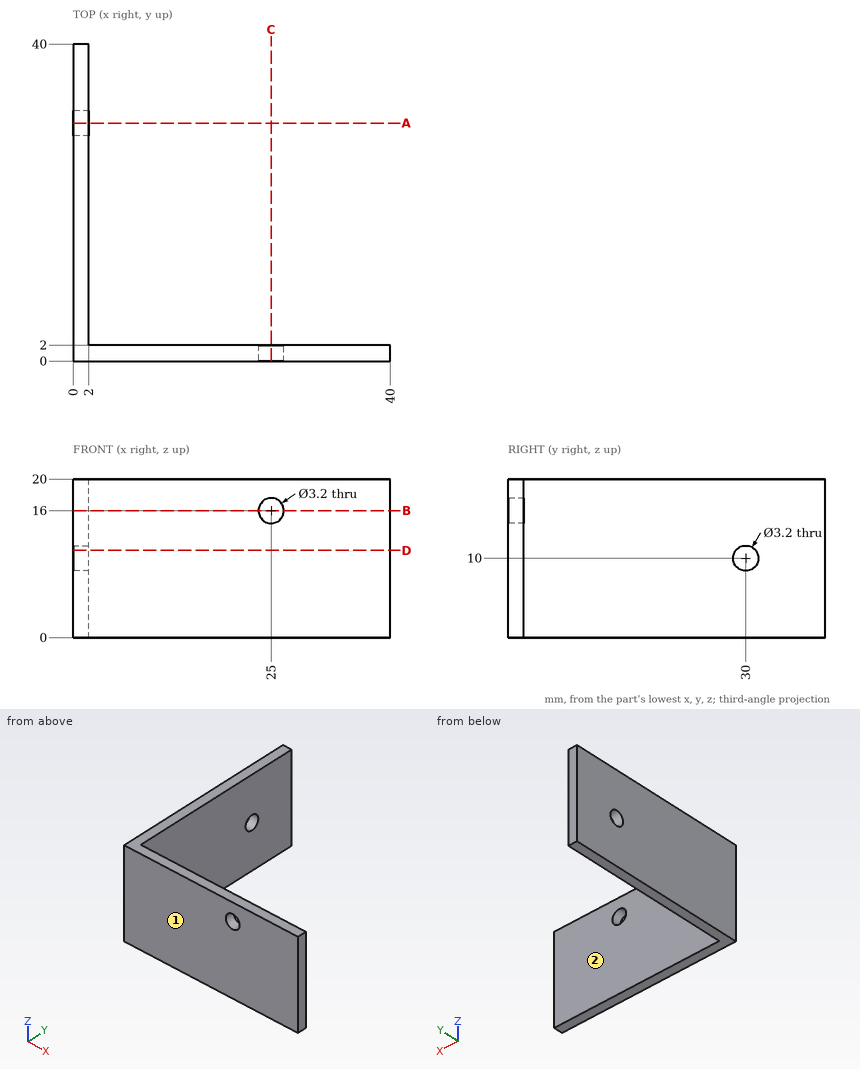
Print and shaded views of the part. All mm, measured from the part's lowest x, y and z. A direction names the side the tool comes from. Give positions to 0.01 mm unless a question says otherwise; leave off trailing zeros. Loops run counter-clockwise (first coordinate to the right, second up) from the corner with the lowest first, then second, coordinate; pieces in that order, holes last. Notation, with made-up numbers: (-17, -11.75) -> (35, -11.75) arc R22 ccw to (35, -0.75) -> close; hole circle Ø3 at (16.5, -10). An arc over 180 degrees is marked (long way). One line per question, with ' | ' between items. Start each with the question number.
1) 3-axis set-ups, long thin cutter, end or side, ignore diameter. For the marked faces 1 and 2: which of +Z, -Z, +X, -X, +Y, -Y reach the whole face in a straight line?
2) Cut at D-D (z = 11). Give the cut face in (x, y), plus the area to 3 significant figures.
3) Pin check, flat tips, straight feed: pin 1 (10 mm diameter, centred on y = 15, z = 5, fed in from +X); pin 2 (8 mm diameter, centred on x = 26, z = 3, fed in from +Y). Stop position of each tip, or through.
4) Cut at B-B (z = 16). Give the cut face in (x, y).
5) Cut at A-A (y = 30). Give the cut face in (x, z), plus the area to 3 significant figures.
6) Cut at C-C (x = 25). Give the cut face in (y, z), plus the area to 3 significant figures.
7) Probe L1, parallel to Z at x = 25, y = 0.95; L2, parallel to Y at x = 0.95, z = 10; L3, parallel to Y at x = 27, z = 18.75. List the from-to ranges inside material, lowest first.
Return value:
1) face 1: +Z, -Z, +X, -X, -Y | face 2: +Z, -Z, +X, +Y
2) outline: (0, 0) -> (40, 0) -> (40, 2) -> (2, 2) -> (2, 28.75) -> (0, 28.75) -> close; (0, 31.25) -> (2, 31.25) -> (2, 40) -> (0, 40) -> close | area: 151 mm^2
3) pin 1: x = 2 | pin 2: y = 2
4) outline: (0, 0) -> (23.4, 0) -> (23.4, 2) -> (2, 2) -> (2, 40) -> (0, 40) -> close; (26.6, 0) -> (40, 0) -> (40, 2) -> (26.6, 2) -> close
5) outline: (0, 0) -> (2, 0) -> (2, 8.4) -> (0, 8.4) -> close; (0, 11.6) -> (2, 11.6) -> (2, 20) -> (0, 20) -> close | area: 33.6 mm^2
6) outline: (0, 0) -> (2, 0) -> (2, 14.4) -> (0, 14.4) -> close; (0, 17.6) -> (2, 17.6) -> (2, 20) -> (0, 20) -> close | area: 33.6 mm^2
7) L1: 0 to 14.4, 17.6 to 20 | L2: 0 to 28.4, 31.6 to 40 | L3: 0 to 2
